Print and shaded views of the part. All mm, measured from the part's lowest x, y and z. Give positions to 0.01 mm unless a question says otherwise; leave off trailing zeros. Loops run counter-clockwise (first coordinate to the right, second up) from the corner with the lowest first, then second, coordinate; pieces in that order, holes last. Notation, with made-up numbers: (-10.75, 76.5) - (22.25, 76.5) arc R13 cw to (22.25, 89.5) - close; hole circle Ø6 at (20.5, 38). An arc over 180 degrees is marked (long way). Return JSON: item names as keys, results as strings.
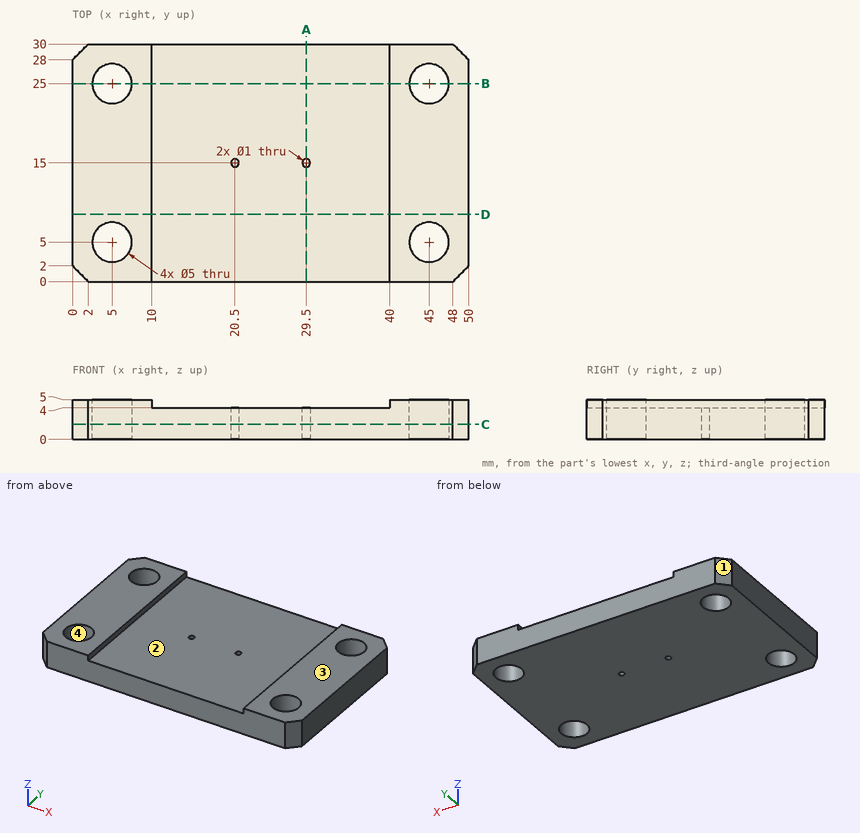
1. Cut at A-A, the plane x = 29.5. Write the cut outline in (y, z), plus the area to 3 significant figures.
Values follow:
{"outline": "(0, 0) - (14.5, 0) - (14.5, 4) - (0, 4) - close; (15.5, 0) - (30, 0) - (30, 4) - (15.5, 4) - close", "area": "116 mm²"}
2. Cut at D-D, the plane y = 8.5. Write the cut outline in (x, z).
Values follow:
{"outline": "(0, 0) - (50, 0) - (50, 5) - (40, 5) - (40, 4) - (10, 4) - (10, 5) - (0, 5) - close"}
3. Cut at B-B, the plane y = 25. Write the cut outline in (x, z).
Values follow:
{"outline": "(0, 0) - (2.5, 0) - (2.5, 5) - (0, 5) - close; (7.5, 0) - (42.5, 0) - (42.5, 5) - (40, 5) - (40, 4) - (10, 4) - (10, 5) - (7.5, 5) - close; (47.5, 0) - (50, 0) - (50, 5) - (47.5, 5) - close"}
4. Drill centre lines: probe 1 along Y at (x, z) = (45, 2.7); probe 2 along Y at (x, z) = (20.5, 1.75); probe 3 along X at (y, z) = (16.75, 4.3). Where is each one in solid material? Low to high.
Values follow:
{"probe 1": "y = 0 to 2.5, 7.5 to 22.5, 27.5 to 30", "probe 2": "y = 0 to 14.5, 15.5 to 30", "probe 3": "x = 0 to 10, 40 to 50"}
5. Pull direction X, two halves, no side cores. Call the marked faces 1, 2, 3 and 4: +X half, -X half, draft (parallel to the pull), parting line (faces both ways), or undercut.
Values follow:
{"face 1": "-X half", "face 2": "undercut", "face 3": "draft", "face 4": "undercut"}
6. Drop a flat-ended pin along its axis: P1, Ø1.5, axis at x = 31.5, y = 9, coming from the +Z side. Give the stop position or say it passes through.
Values follow:
{"P1": "stops at z = 4"}
7. Cut at C-C, the plane z = 1.9. Write the cut outline in (x, y).
Values follow:
{"outline": "(0, 2) - (2, 0) - (48, 0) - (50, 2) - (50, 28) - (48, 30) - (2, 30) - (0, 28) - close; hole circle Ø5 at (5, 5); hole circle Ø5 at (5, 25); hole circle Ø1 at (20.5, 15); hole circle Ø1 at (29.5, 15); hole circle Ø5 at (45, 5); hole circle Ø5 at (45, 25)"}
